Can you work these out from the model? Positions are in its coordinate system, mm. A direction names the side the tool comes from. Give positions to 0.01 mm unless a question says otherwise; leave off trailing zeros. Order: outer loops, then holes, each group sorted by start corner. A loop starts at its lowest first (then second) coordinate and runs counter-clockwise, first axis right, second up. Notation, with made-up numbers: (36, -27) -> (48, -27) arc R25 ccw to (48, 7) -> close; hole circle Ø11 at (38, -13). An arc over 180 degrees is marked (long way). Answer as a JSON object with one key per item and string values.
```python
from build123d import *

# Parameters (mm, degrees)
BOSS_EXTRUDE1_DEPTH = 550
SKETCH2_R           = 1.55
CUT_EXTRUDE1_DEPTH  = 10
SKETCH3_R           = 1.55
CUT_EXTRUDE2_DEPTH  = 10


with BuildPart() as part:
    # Sketch1 → Boss-Extrude1 (new body)
    with BuildSketch(Plane.XY):
        Polygon((0, 0), (0, 25), (1.5, 25), (1.5, 1.5), (25, 1.5), (25, 0), align=None)
    extrude(amount=BOSS_EXTRUDE1_DEPTH)

    # Sketch2 → Cut-Extrude1 (cut)
    with BuildSketch(Plane.ZY):
        with Locations((10, 10)):
            Circle(SKETCH2_R)
        with Locations((20, 20)):
            Circle(SKETCH2_R)
        with Locations((530, 20)):
            Circle(SKETCH2_R)
        with Locations((540, 10)):
            Circle(SKETCH2_R)
    extrude(amount=-CUT_EXTRUDE1_DEPTH, mode=Mode.SUBTRACT)

    # Sketch3 → Cut-Extrude2 (cut)
    with BuildSketch(Plane.XZ):
        with Locations((10, 540)):
            Circle(SKETCH3_R)
        with Locations((20, 530)):
            Circle(SKETCH3_R)
        with Locations((20, 20)):
            Circle(SKETCH3_R)
        with Locations((10, 10)):
            Circle(SKETCH3_R)
    extrude(amount=-CUT_EXTRUDE2_DEPTH, mode=Mode.SUBTRACT)


solid = part.part
```
1. Will this pin go through, and if not, where does the flat tip stop? pin 1 Ø1.5 at (x, z) = (10, 142.5) entering from +Y.
Worked answers:
{"pin 1": "y = 1.5"}
2. If we section it at A-A on z = 117: Please give me the cut outline in (x, y).
Worked answers:
{"outline": "(0, 0) -> (25, 0) -> (25, 1.5) -> (1.5, 1.5) -> (1.5, 25) -> (0, 25) -> close"}
3. For faces 1 (the face through (13, 0, 271)), 2 (the face through (1.5, 13, 271)), which set-ups out of +Z, -Z, +X, -X, +Y, -Y let a thin tool reach every point of the face, with its end or its side?
Worked answers:
{"face 1": "+Z, -Z, +X, -X, -Y", "face 2": "+Z, -Z, +X, +Y"}
4. Please list where these lines run through material, in increasing order: L1, parallel to Y at x = 1.2, z = 540; L2, parallel to Z at x = 10, y = 0.5; L3, parallel to Y at x = 1.2, z = 20.
Worked answers:
{"L1": "0 to 8.45, 11.55 to 25", "L2": "0 to 8.45, 11.55 to 538.45, 541.55 to 550", "L3": "0 to 18.45, 21.55 to 25"}
